Could you check a few things on this model? Use its own coordinates, in mm. A direction names the side the tool comes from. Give positions to 0.01 mm unless a question says otherwise; leave off trailing zeros. Write each loop counter-clockwise with the first axis right and the second up, starting at its lowest first coordinate (ties: lowest second). Pieces come first, ordered by that corner, then holes. Notation, with made-up numbers: M 66,34.5 L 100,34.5 A28 ccw 100,52.5 Z; hole C 16.5,-4.75 d1. An arc over 180 degrees is marked long. Write each question's results on one line, items separated by ' | '. Start each with the question number.
from build123d import *

# Parameters (mm, degrees)
SKETCH2_R           = 2.6
CORE_DEPTH          = 11
SKETCH5_W           = 9.1
SKETCH5_H           = 3.5
HEX_NUT_DEPTH       = 14.2
BOLT_GUARD_DEPTH    = 2
SKETCH7_R           = 2.6
D_SHAFT_DEPTH       = 15
SKETCH8_R           = 3
SET_SCREW_DEPTH     = 35.195516275
BOSS_EXTRUDE1_REACH = 27.116


with BuildPart() as part:
    # Sketch2 → core (new body)
    with BuildSketch(Plane(origin=(0, 0, 0), x_dir=(1, 0, 0), z_dir=(0, 1, 0))):
        Polygon((9.814954576, 0), (4.907477288, 8.5), (-4.907477288, 8.5), (-9.814954576, 0), (-4.907477288, -8.5), (4.907477288, -8.5), align=None)
        with Locations(Location((0, 0, 0), (0, 0, 270))):
            Circle(SKETCH2_R, mode=Mode.SUBTRACT)
    extrude(amount=CORE_DEPTH)

    # Sketch5 → hex-nut (cut)
    with BuildSketch(Plane.XY.offset(8.5)):
        with Locations((0, 4.75)):
            Rectangle(SKETCH5_W, SKETCH5_H)
    extrude(amount=-HEX_NUT_DEPTH, mode=Mode.SUBTRACT)

    # Sketch4 → bolt-guard (add)
    with BuildSketch(Plane(origin=(0, 11, 0), x_dir=(1, 0, 0), z_dir=(0, 1, 0))):
        Polygon((9.814954576, 0), (4.907477288, 8.5), (-4.907477288, 8.5), (-9.814954576, 0), (-4.907477288, -8.5), (4.907477288, -8.5), align=None)
    extrude(amount=BOLT_GUARD_DEPTH)

    # Sketch7 → d-shaft (add)
    with BuildSketch(Plane(origin=(0, 13, 0), x_dir=(1, 0, 0), z_dir=(0, 1, 0))):
        Polygon((9.814954576, 0), (4.907477288, 8.5), (-4.907477288, 8.5), (-9.814954576, 0), (-4.907477288, -8.5), (4.907477288, -8.5), align=None)
        Circle(SKETCH7_R, mode=Mode.SUBTRACT)
    extrude(amount=D_SHAFT_DEPTH)

    # Sketch8 → set-screw (cut, through all)
    with BuildSketch(Plane.XY.offset(8.5)):
        with Locations((0, 23.5)):
            Circle(SKETCH8_R)
    extrude(amount=-SET_SCREW_DEPTH, mode=Mode.SUBTRACT)

    # Sketch9 → Boss-Extrude1 (add, up to next)
    with BuildSketch(Plane.XZ.offset(-6.5), mode=Mode.PRIVATE) as boss_extrude1_sk1:
        Polygon((4.55, -5.7), (4.55, 0), (2.275, -3.940415587), (-2.275, -3.940415587), (-4.55, 0), (-4.55, -5.7), align=None)
    boss_extrude1_tool1 = extrude(boss_extrude1_sk1.sketch, amount=BOSS_EXTRUDE1_REACH, mode=Mode.PRIVATE) - part.part
    add(boss_extrude1_tool1.solids().sort_by_distance((0, 6.5, -4.033017))[0])


solid = part.part
Q1. I'm going to push flat-ended pins straight in: P1, Ø4, axis at x = 0, z = 0, coming from the +Y side; P2, Ø5.5, axis at x = 0, y = 23.5, coming from the +Z side; P3, Ø1.8, axis at y = 5.5, z = 2, coming from the -X side; P4, Ø4, axis at y = 4, z = 5.5, coming from the +X side. Where does each tip first touch, or does it pass through?
Q2. If we section it at C-C (y = 17.5): Please give me the cut outline in (x, z).
Q3. If we mould it in two halves opening along Z, with no side actions, what happens to faces 1 (the face through (4.55, 5, 4)), 2 (the face through (7.396, 13.804, -4.191)), 3 (the face through (0, 11, 0))? For each: pulls with the +Z half, pulls with the -Z half, needs draft (parallel to the pull), parting line crosses it, or undercut.
Q4. If we section it at B-B (x = 0): Please give me the cut outline in (y, z), plus the area to 3 significant figures.
Q5. If we section it at D-D (z = 5.75): Please give me the cut outline in (x, y), plus the area to 3 significant figures.
Q6. For faces 4 (the face through (0.78, 8.72, 2.48)), 5 (the face through (0, 5, -3.94)), 6 (the face through (0, 13, 0)), which set-ups out of +Z, -Z, +X, -X, +Y, -Y let a thin tool reach every point of the face, with its end or its side?
Q7. Please list where these lines run through material, in increasing order: line 1 (Y direction, x = 0, z = -3); line 2 (Z direction, x = 0, y = 2.3); line 3 (Y direction, x = -1, z = 7.25). Write a range as [from, to].
Q8. If we section it at A-A (y = 23.5): Please give me the cut outline in (x, z), plus the area to 3 significant figures.
Determined:
1) P1: stops at y = 13 | P2: passes through | P3: stops at x = -9.18 | P4: stops at x = 7.79
2) outline: M -9.81,0 L -4.91,-8.5 L 4.91,-8.5 L 9.81,0 L 4.91,8.5 L -4.91,8.5 Z; hole C 0,0 d5.2
3) face 1: needs draft | face 2: pulls with the -Z half | face 3: undercut
4) outline: M 0,-8.5 L 20.5,-8.5 L 20.5,-2.6 L 13,-2.6 L 13,2.6 L 20.5,2.6 L 20.5,8.5 L 6.5,8.5 L 6.5,2.6 L 11,2.6 L 11,-2.6 L 6.5,-2.6 L 6.5,-3.94 L 3,-3.94 L 3,-2.6 L 0,-2.6 Z; M 0,2.6 L 3,2.6 L 3,8.5 L 0,8.5 Z; M 26.5,-8.5 L 28,-8.5 L 28,-2.6 L 26.5,-2.6 Z; M 26.5,2.6 L 28,2.6 L 28,8.5 L 26.5,8.5 Z | area: 245 mm²
5) outline: M -6.5,0 L 6.5,0 L 6.5,28 L -6.5,28 Z; hole M -4.55,3 L 4.55,3 L 4.55,6.5 L -4.55,6.5 Z; hole C 0,23.5 d6 | area: 304 mm²
6) face 4: -Y | face 5: +Z | face 6: +Y
7) line 1: y = [0, 3], [6.5, 20.5], [26.5, 28] | line 2: z = [-8.5, -2.6], [2.6, 8.5] | line 3: y = [0, 3], [6.5, 20.67], [26.33, 28]
8) outline: M -9.81,0 L -4.91,-8.5 L -3,-8.5 L -3,8.5 L -4.91,8.5 Z; M 3,-8.5 L 4.91,-8.5 L 9.81,0 L 4.91,8.5 L 3,8.5 Z | area: 148 mm²
